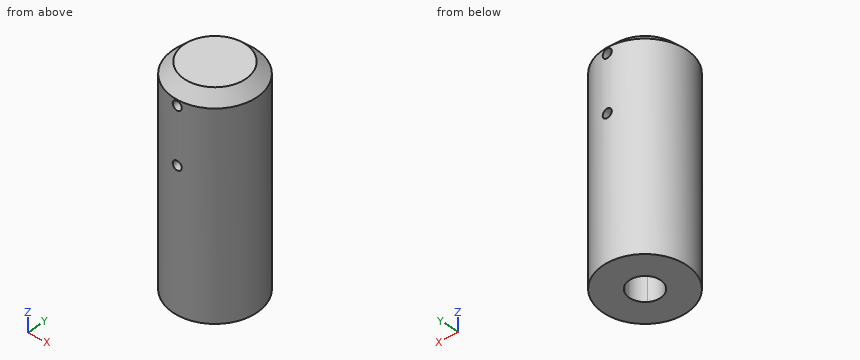
```python
from build123d import *

# Parameters (mm, degrees)
F0_R     = 7.5
F1_DEPTH = 38
F3_R     = 0.8
F4_DEPTH = 15.001
F5_SIZE  = 2
F7_DEPTH = 23
F8_DEPTH = 7


with BuildPart() as f1:
    # F0 (on Top) → F1 (new body)
    with BuildSketch(Plane.XY):
        Circle(F0_R)
    extrude(amount=F1_DEPTH)

    # F3 (on offset) → F4 (cut, through all)
    with BuildSketch(Plane.XZ.offset(7.5)):
        with Locations((0, 35)):
            Circle(F3_R)
        with Locations((0, 25)):
            Circle(F3_R)
    extrude(amount=-F4_DEPTH, mode=Mode.SUBTRACT)

    # F5
    f5_edges = [f1.edges().sort_by_distance(p)[0] for p in [
        (-7.5, 0, 38),
    ]]
    chamfer(f5_edges, length=F5_SIZE)

    # F6 (on face) → F7 (cut)
    with BuildSketch(Plane(origin=(0, 0, 0), x_dir=(1, 0, 0), z_dir=(0, 0, -1))):
        with BuildLine():
            ThreePointArc((-1.596872, 2.3), (-1.297836, -2.481052), (2.8, 0))
            ThreePointArc((2.8, 0), (2.481052, 1.297836), (1.596872, 2.3))
            Line((1.596872, 2.3), (-1.596872, 2.3))
        make_face()
    extrude(amount=-F7_DEPTH, mode=Mode.SUBTRACT)

    # F6 (on face) → F8 (cut)
    with BuildSketch(Plane(origin=(0, 0, 0), x_dir=(1, 0, 0), z_dir=(0, 0, -1))):
        with BuildLine():
            Line((-1.596872, 2.3), (1.596872, 2.3))
            ThreePointArc((1.596872, 2.3), (0, 2.8), (-1.596872, 2.3))
        make_face()
    extrude(amount=-F8_DEPTH, mode=Mode.SUBTRACT)


solid = f1.part
```
For this review, take the finished solid that the model builds, in its own axes (mm). Coordinates: 2 decimals unless noted, no trailing zeros. Loops run counter-clockwise (first coordinate to the right, second up) from the corner with the lowest first, then second, coordinate; pieces in that order, holes last.
1. Insertion check: P1, Ø4.5, axis at x = 0, y = 0, coming from the -Z side; P2, Ø1, axis at y = -3, z = 26, coming from the +X side; P3, Ø2, axis at x = -3.5, z = 29, coming from the -Y side. Each pin has a flat end and moves straight along its axis. Give the tip position at first contact, or say it passes through.
2. Add section C-C, the plane z = 30. Give the boundary of the cut face in (x, y).
3. Add section B-B, the plane y = 4. Count the separate pieces of the cut face and the enclosed holes in it, then the cut area to 3 significant figures.
4. Add section A-A, the plane z = 18. Give the boundary of the cut face in (x, y), then the cut area to 3 significant figures.
5. For line 1 (Z direction, x = 0, y = 0.5); line 2 (Z direction, x = 0, y = 4.25); line 3 (Y direction, x = 0, z = 12.25), list the stretches that pass through material, from the lowest coordinate up.
6. Add section D-D, the plane z = 3. Give the boundary of the cut face in (x, y).
Result:
1. P1: stops at z = 23
1. P2: stops at x = 7.07
1. P3: stops at y = -7.07
2. outline: circle Ø15 at (0, 0)
3. separate pieces: 1
3. enclosed holes: 2
3. area: 473 mm2
4. outline: circle Ø15 at (0, 0); hole (-1.6, -2.3) - (1.6, -2.3) arc R2.8 ccw to (2.8, 0) arc R2.8 ccw (long way) to start
4. area: 153 mm2
5. line 1: z = 23 to 24.2, 25.8 to 34.2, 35.8 to 38
5. line 2: z = 0 to 24.2, 25.8 to 34.2, 35.8 to 38
5. line 3: y = -7.5 to -2.3, 2.8 to 7.5
6. outline: circle Ø15 at (0, 0); hole (1.6, -2.3) arc R2.8 ccw to (2.8, 0) arc R2.8 ccw (long way) to start
